Study the drawing (mm; zero at the part's minimum x, y, z) and answer. Give positions to 0.01 mm unless a question says otherwise; leave off trailing zeros. Loops run counter-clockwise (first coordinate to the right, second up) from the corner with the lowest first, then second, coordinate; pieces in that order, holes last. Notation, with made-up numbers: (4, -39) - (42, -39) arc R10 cw to (42, -22) - close; hole circle Ø9 at (28.5, -22.5). An arc over 180 degrees is marked (long way). Write item = value, one per line. Start each with the question number.
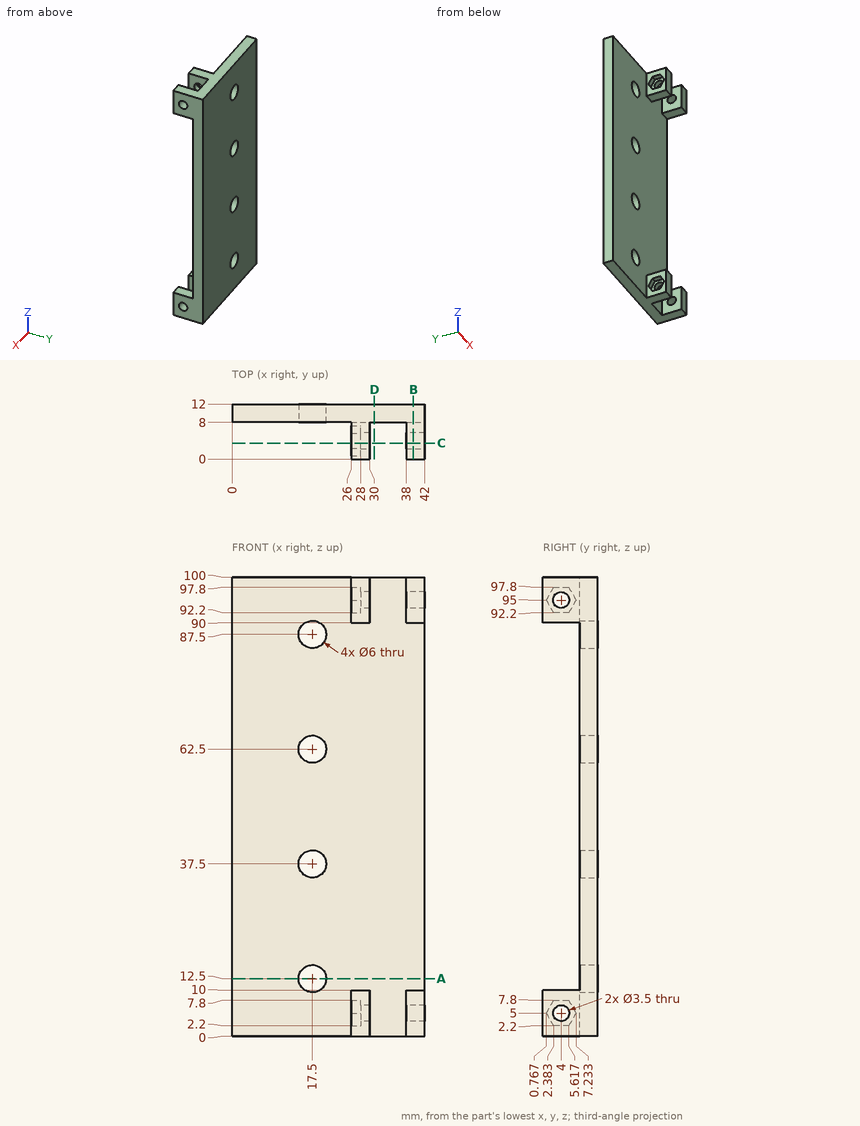
1. Given P1, Ø1, axis at x = 14.5, z = 17, coming from the -Y side; P2, Ø5, axis at y = 8, z = 28, coming from the -X side; P3, Ø3, axis at y = 4, z = 95, coming from the +X side; P4, Ø2.5, axis at y = 6, z = 92.5, coming from the -X side, each flat-ended and moving along its own axis, determine where each tip first touches the part or whether it passes through.
2. A cutting plane is placed at D-D on x = 31. Give the vertices of the cut face in (y, z).
3. A cutting plane is placed at A-A on z = 12.5. Give the vertices of the cut face in (x, y), and give its area (3 significant figures).
4. A cutting plane is placed at B-B on x = 39.5. Give the vertices of the cut face in (y, z).
5. Consider line 1 along Z through (x, y) = (17.5, 8.75); line 2 along Z through (x, y) = (39.95, 4); line 3 along Y through (x, z) = (38, 47). Determine where each line is inside the solid, lowest interval first. Write a range as [from, to].
6. A cutting plane is placed at C-C on y = 3.5. Give the number of separate pieces and of enclosed holes in the cut face.
Reply:
q1.P1 = 8
q1.P2 = 0
q1.P3 = through
q1.P4 = 26
q2.outline = (8, 0) - (12, 0) - (12, 100) - (8, 100) - close
q3.outline = (0, 8) - (14.5, 8) - (14.5, 12) - (0, 12) - close; (20.5, 8) - (42, 8) - (42, 12) - (20.5, 12) - close
q3.area = 144 mm^2
q4.outline = (0, 0) - (12, 0) - (12, 100) - (0, 100) - (0, 90) - (8, 90) - (8, 10) - (0, 10) - close; hole circle Ø3.5 at (4, 5); hole circle Ø3.5 at (4, 95)
q5.line_1 = [0, 9.5], [15.5, 34.5], [40.5, 59.5], [65.5, 84.5], [90.5, 100]
q5.line_2 = [0, 3.25], [6.75, 10], [90, 93.25], [96.75, 100]
q5.line_3 = [8, 12]
q6.separate_pieces = 8
q6.enclosed_holes = 0
